Part print with two shaded views. Sizes in mm from the minimum x, y, z corner. A direction names the side the tool comes from. Round coordinates to 2 decimals unless told otherwise and drop trailing zeros. Order: outer loops, then holes, each group sorted by start corner. A loop starts at its lowest first (then second) coordinate and runs counter-clockwise, first axis right, second up. Notation, with made-up numbers: (73.5, -2) -> (121.5, -2) arc R26 cw to (121.5, 12) -> close; hole circle Ø1 at (56, -8). An arc over 180 degrees is marked (long way). Answer as a JSON object with one key per item and string values.
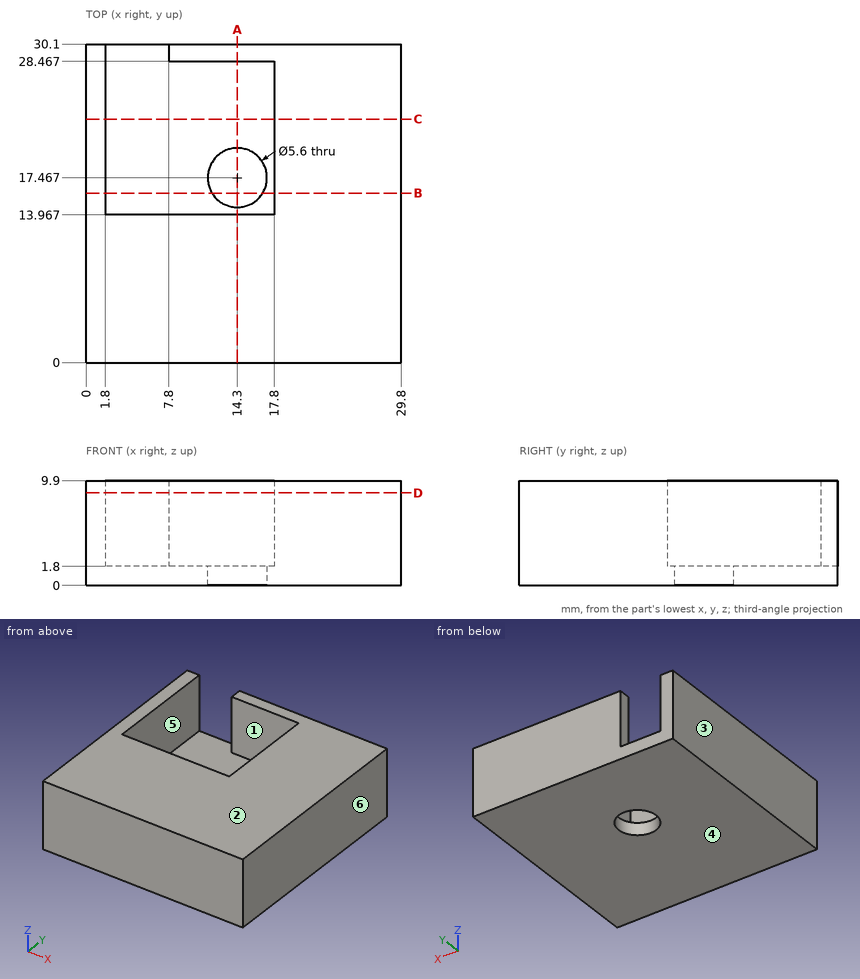
1) Which spindle directions (+Z, -Z, +X, -X, +Y, -Y) get a long thin tool onto all of the face, cutting with end or side? Do the marked faces 1 and 2. Say none if no direction does.
Checked values:
{"face 1": "+Z", "face 2": "+Z, +X, -X, +Y, -Y"}
2) Pull direction X, two halves, no side cores. Call the marked faces 3, 4, 5 and 6: pulls with the +X half, pulls with the -X half, needs draft (parallel to the pull), parting line crosses it, or undercut.
Checked values:
{"face 3": "pulls with the -X half", "face 4": "needs draft", "face 5": "undercut", "face 6": "pulls with the +X half"}
3) Cut at D-D, the plane z = 8.75. Give the cut face in (x, y), plus the area to 3 significant figures.
Checked values:
{"outline": "(0, 0) -> (29.8, 0) -> (29.8, 30.1) -> (7.8, 30.1) -> (7.8, 28.47) -> (17.8, 28.47) -> (17.8, 13.97) -> (1.8, 13.97) -> (1.8, 30.1) -> (0, 30.1) -> close", "area": "655 mm²"}
4) Cut at B-B, the plane y = 16. Give the cut face in (x, z) (3 decimals).
Checked values:
{"outline": "(0, 0) -> (11.915, 0) -> (11.915, 1.8) -> (1.8, 1.8) -> (1.8, 9.9) -> (0, 9.9) -> close; (16.685, 0) -> (29.8, 0) -> (29.8, 9.9) -> (17.8, 9.9) -> (17.8, 1.8) -> (16.685, 1.8) -> close"}
5) Cut at C-C, the plane y = 23. Give the cut face in (x, z).
Checked values:
{"outline": "(0, 0) -> (29.8, 0) -> (29.8, 9.9) -> (17.8, 9.9) -> (17.8, 1.8) -> (1.8, 1.8) -> (1.8, 9.9) -> (0, 9.9) -> close"}
6) Flat gauge pin, fed straight in: pin 1 Ø5 at (x, y) = (10.5, 25) entering from +Z. Where does the tip first touch, or does it go through?
Checked values:
{"pin 1": "stops at z = 1.8"}
7) Cut at A-A, the plane x = 14.3. Give the cut face in (y, z).
Checked values:
{"outline": "(0, 0) -> (14.67, 0) -> (14.67, 1.8) -> (13.97, 1.8) -> (13.97, 9.9) -> (0, 9.9) -> close; (20.27, 0) -> (30.1, 0) -> (30.1, 9.9) -> (28.47, 9.9) -> (28.47, 1.8) -> (20.27, 1.8) -> close"}
8) Probe L1, parallel to Y at x = 12.75, z = 5.5; L2, parallel to Y at x = 14.3, z = 1.2; L3, parallel to X at y = 17.5, z = 5.75. List the from-to ranges inside material, lowest first. Write a range as from..to.
Checked values:
{"L1": "y = 0..13.97, 28.47..30.1", "L2": "y = 0..14.67, 20.27..30.1", "L3": "x = 0..1.8, 17.8..29.8"}
